from build123d import *

# Parameters (mm, degrees)
SKETCH1_W           = 108.4
SKETCH1_H           = 72
BOSS_EXTRUDE1_DEPTH = 10
SKETCH2_W           = 93
SKETCH2_H           = 56.6
CUT_EXTRUDE1_DEPTH  = 131.516512365
SKETCH4_W           = 6
SKETCH4_H           = 6
BOSS_EXTRUDE2_DEPTH = 6.35
SKETCH5_W           = 6
SKETCH5_H           = 6
BOSS_EXTRUDE3_DEPTH = 6.35
SKETCH6_W           = 6
SKETCH6_H           = 6
BOSS_EXTRUDE4_DEPTH = 6.35
SKETCH7_W           = 6
SKETCH7_H           = 6
BOSS_EXTRUDE5_DEPTH = 6.35


with BuildPart() as part:
    # Sketch1 → Boss-Extrude1 (new body)
    with BuildSketch(Plane(origin=(0, 0, 0), x_dir=(1, 0, 0), z_dir=(0, 1, 0))):
        with Locations((54.2, 36)):
            Rectangle(SKETCH1_W, SKETCH1_H)
    extrude(amount=BOSS_EXTRUDE1_DEPTH)

    # Sketch2 → Cut-Extrude1 (cut, through all)
    with BuildSketch(Plane(origin=(0, 10, 0), x_dir=(1, 0, 0), z_dir=(0, 1, 0))):
        with Locations((54.2, 36)):
            Rectangle(SKETCH2_W, SKETCH2_H)
    extrude(amount=-CUT_EXTRUDE1_DEPTH, mode=Mode.SUBTRACT)

    # Sketch4 → Boss-Extrude2 (add)
    with BuildSketch(Plane(origin=(0, 10, 0), x_dir=(1, 0, 0), z_dir=(0, 1, 0))):
        with Locations((4, 4)):
            Rectangle(SKETCH4_W, SKETCH4_H)
    extrude(amount=BOSS_EXTRUDE2_DEPTH)

    # Sketch5 → Boss-Extrude3 (add)
    with BuildSketch(Plane(origin=(0, 10, 0), x_dir=(1, 0, 0), z_dir=(0, 1, 0))):
        with Locations((104.4, 4)):
            Rectangle(SKETCH5_W, SKETCH5_H)
    extrude(amount=BOSS_EXTRUDE3_DEPTH)

    # Sketch6 → Boss-Extrude4 (add)
    with BuildSketch(Plane(origin=(0, 10, 0), x_dir=(1, 0, 0), z_dir=(0, 1, 0))):
        with Locations((4, 68)):
            Rectangle(SKETCH6_W, SKETCH6_H)
    extrude(amount=BOSS_EXTRUDE4_DEPTH)

    # Sketch7 → Boss-Extrude5 (add)
    with BuildSketch(Plane(origin=(0, 10, 0), x_dir=(1, 0, 0), z_dir=(0, 1, 0))):
        with Locations((104.4, 68)):
            Rectangle(SKETCH7_W, SKETCH7_H)
    extrude(amount=BOSS_EXTRUDE5_DEPTH)


solid = part.part
Verification items for the finished model (mm, model axes). A direction names the side the tool comes from. Coordinates: 2 decimals unless noted, no trailing zeros. Write each loop counter-clockwise with the first axis right and the second up, starting at its lowest first coordinate (ties: lowest second). Pieces come first, ordered by that corner, then holes. Notation, with made-up numbers: M 79.5,63.25 L 120.5,63.25 A22 ccw 120.5,97.25 Z; hole C 13.25,51.5 d3. An arc over 180 degrees is marked long. Use a Markdown table: item, result.
Q1. Thickness scan on line 1 (Z direction, x = 41, y = 6); line 2 (X direction, y = 3.5, z = -36.5); line 3 (X direction, y = 15, z = -66). Record the ranges inside material, lowest first.
Reply:
| item | result |
|---|---|
| line 1 | z = -72 to -64.3, -7.7 to 0 |
| line 2 | x = 0 to 7.7, 100.7 to 108.4 |
| line 3 | x = 1 to 7, 101.4 to 107.4 |
Q2. Sectioned sample at C-C, the plane y = 6.5. Record the boundary of the cut face in (x, z).
Reply:
| item | result |
|---|---|
| outline | M 0,-72 L 108.4,-72 L 108.4,0 L 0,0 Z; hole M 7.7,-64.3 L 100.7,-64.3 L 100.7,-7.7 L 7.7,-7.7 Z |
Q3. Sectioned sample at A-A, the plane x = 72.5. Record the boundary of the cut face in (y, z).
Reply:
| item | result |
|---|---|
| outline | M 0,-72 L 10,-72 L 10,-64.3 L 0,-64.3 Z; M 0,-7.7 L 10,-7.7 L 10,0 L 0,0 Z |
Q4. Sectioned sample at D-D, the plane z = -4.5. Record the boundary of the cut face in (x, y), plus the area to 3 significant figures.
Reply:
| item | result |
|---|---|
| outline | M 0,0 L 108.4,0 L 108.4,10 L 107.4,10 L 107.4,16.35 L 101.4,16.35 L 101.4,10 L 7,10 L 7,16.35 L 1,16.35 L 1,10 L 0,10 Z |
| area | 1,160 mm² |
Q5. Draft check along Z on faces 1 (the face through (54, 5, -7.7)), 2 (the face through (7, 13, -68)), 3 (the face through (104, 13, -1)). Enter one of: +Z half, -Z half, draft (parallel to the pull), parting line (faces both ways), or undercut.
Reply:
| item | result |
|---|---|
| face 1 | undercut |
| face 2 | draft |
| face 3 | +Z half |
Q6. Go/stop test with flat-tipped pins: P1, Ø5, axis at y = 14.5, z = -68, coming from the -X side; P2, Ø5, axis at x = 4.5, y = 13.5, coming from the +Z side; P3, Ø6, axis at x = 11, z = -32.5, coming from the -Y side; P4, Ø6, axis at x = 71, y = 10, coming from the +Z side. Record where each tip stops, or that it passes through.
Reply:
| item | result |
|---|---|
| P1 | stops at x = 1 |
| P2 | stops at z = -1 |
| P3 | passes through |
| P4 | stops at z = 0 |
Q7. Set-up check for faces 4 (the face through (104, 13, -7)), 5 (the face through (54, 5, -64.3)), 6 (the face through (101.4, 13, -4)): record each of +Z, -Z, +X, -X, +Y, -Y from which the full face is reachable in a straight line by a thin tool's end or side.
Reply:
| item | result |
|---|---|
| face 4 | +X, -X, +Y |
| face 5 | +Y, -Y |
| face 6 | +Z, -Z, +Y |
Q8. Sectioned sample at B-B, the plane z = -30. Record the boundary of the cut face in (x, y).
Reply:
| item | result |
|---|---|
| outline | M 0,0 L 7.7,0 L 7.7,10 L 0,10 Z; M 100.7,0 L 108.4,0 L 108.4,10 L 100.7,10 Z |
